```python
from build123d import *

# Parameters (mm, degrees)
CROQUIS1_RX                = 6.036526162
CROQUIS1_RY                = 3.070539463
CROQUIS1_RX_2              = 3.326417752
CROQUIS1_RY_2              = 2.687947262
SALIENTE_EXTRUIR2_DEPTH    = 5
CROQUIS7_W                 = 42.690533415
CROQUIS7_H                 = 0.890099334
CORTAR_EXTRUIR1_DEPTH      = 10
REDONDEO1_R                = 2.5
CROQUIS3_R                 = 1.1
SALIENTE_EXTRUIR3_DEPTH    = 11.5
SALIENTE_EXTRUIR4_START    = 11.5
CROQUIS6_R                 = 1.1
SALIENTE_EXTRUIR4_DEPTH    = 11.5
CORTAR_EXTRUIR2_DEPTH      = 61.024571756
CORTAR_EXTRUIR2_DEPTH_BACK = 61.024571756


with BuildPart() as part:
    # Croquis1 → Saliente-Extruir2 (new body)
    with BuildSketch(Plane.YZ):
        with BuildLine():
            Line((20.084653921, 11.717525193), (24.641633022, 14.68917463))
            ThreePointArc((24.641633022, 14.68917463), (27.816291871, 14.320547257), (28.034373421, 11.132007562))
            Line((28.034373421, 11.132007562), (20, 0))
            Line((20, 0), (20, -10))
            Line((20, -10), (15, -10))
            Line((15, -10), (15, -4.5))
            Line((15, -4.5), (3.5, -4.5))
            Line((3.5, -4.5), (3.5, -10))
            Line((3.5, -10), (-3.5, -10))
            Line((-3.5, -10), (-3.5, -4.5))
            Line((-3.5, -4.5), (-15, -4.5))
            Line((-15, -4.5), (-15, -10))
            Line((-15, -10), (-20, -10))
            Line((-20, -10), (-20, 0))
            Line((-20, 0), (-28.034373421, 11.132007562))
            ThreePointArc((-28.034373421, 11.132007562), (-27.816291871, 14.320547257), (-24.641633022, 14.68917463))
            Line((-24.641633022, 14.68917463), (-20.084653921, 11.717525193))
            ThreePointArc((-20.084653921, 11.717525193), (-14.865648019, 27.519606107), (0, 35))
            ThreePointArc((0, 35), (14.865648019, 27.519606107), (20.084653921, 11.717525193))
        make_face()
        with Locations(Location((-8.99716125, 20.68522558), (0, 0, 90))):
            Ellipse(CROQUIS1_RX, CROQUIS1_RY, mode=Mode.SUBTRACT)
        with Locations(Location((0, 6.95309076), (0, 0, -90))):
            Ellipse(CROQUIS1_RX_2, CROQUIS1_RY_2, mode=Mode.SUBTRACT)
        with Locations(Location((8.99716125, 20.68522558), (0, 0, 90))):
            Ellipse(CROQUIS1_RX, CROQUIS1_RY, mode=Mode.SUBTRACT)
    extrude(amount=SALIENTE_EXTRUIR2_DEPTH)

    # Croquis7 → Cortar-Extruir1 (cut)
    with BuildSketch(Plane.YZ):
        with Locations((-0.646243402, -10.047083115)):
            Rectangle(CROQUIS7_W, CROQUIS7_H)
    extrude(amount=CORTAR_EXTRUIR1_DEPTH, mode=Mode.SUBTRACT)

    # Redondeo1
    redondeo1_edges = [part.edges().sort_by_distance(p)[0] for p in [
        (0, 17.5, -9.602033448),
        (5, 17.5, -9.602033448),
        (0, 0, -9.602033448),
        (5, 0, -9.602033448),
        (0, -17.5, -9.602033448),
        (5, -17.5, -9.602033448),
    ]]
    fillet(redondeo1_edges, radius=REDONDEO1_R - 0.0001)  # a hair under: the kernel refuses the full size

    # Croquis3 → Saliente-Extruir3 (add)
    with BuildSketch(Plane(origin=(0, 3.5, 0), x_dir=(-1, 0, 0), z_dir=(0, 1, 0))):
        with Locations(Location((-2.5, -7.45, 0), (0, 0, 270))):
            Circle(CROQUIS3_R)
    extrude(amount=SALIENTE_EXTRUIR3_DEPTH)

    # Croquis6 → Saliente-Extruir4 (add)
    with BuildSketch(Plane.XZ.offset(3.5).offset(SALIENTE_EXTRUIR4_START)):
        with Locations(Location((2.5, -7.45, 0), (0, 0, 270))):
            Circle(CROQUIS6_R)
    extrude(amount=-SALIENTE_EXTRUIR4_DEPTH)

    # Croquis8 → Cortar-Extruir2 (cut, two sides: drawn at the far end of the back side and taken through both)
    with BuildSketch(Plane(origin=(0, 20, 0), x_dir=(-1, 0, 0), z_dir=(0, 1, 0)).offset(-CORTAR_EXTRUIR2_DEPTH_BACK)):
        with BuildLine():
            Line((-74.782541857, 59.609037795), (-6.886174559, -6.99410531))
            ThreePointArc((-6.886174559, -6.99410531), (-2.511263824, -8.781661023), (1.863646912, -6.99410531))
            Line((1.863646912, -6.99410531), (69.76001421, 59.609037795))
            Line((69.76001421, 59.609037795), (69.76001421, -130.610786238))
            Line((69.76001421, -130.610786238), (-74.782541857, -130.610786238))
            Line((-74.782541857, -130.610786238), (-74.782541857, 59.609037795))
        make_face()
    extrude(amount=CORTAR_EXTRUIR2_DEPTH + CORTAR_EXTRUIR2_DEPTH_BACK, mode=Mode.SUBTRACT)


solid = part.part
```
Build history of the part. All positions in model axes, mm. A direction names the side the tool comes from. Round coordinates to 2 decimals unless told otherwise and drop trailing zeros. Loops run counter-clockwise (first coordinate to the right, second up) from the corner with the lowest first, then second, coordinate; pieces in that order, holes last.
Item 1: Two-plate mould, pull along Y, no slides. Class faces 1 (the face through (2.46, 22.33, 13.18)), 2 (the face through (0, 0, 14)), 3 (the face through (2.46, -23.96, 5.49)), 4 (the face through (2, -9, -4.5)): released by +Y, released by -Y, zero draft, split by the parting line, or undercut.
Item 2: Saw through at C-C (y = -18). List the corners of the cut face in (x, z).
Item 3: Drill centre lines: line 1 along Y through (x, z) = (4.6, 16); line 2 along Z through (x, y) = (3.45, 10); line 3 along Y through (x, z) = (0.95, 21.5). Where is each one in solid material? Low to high.
Item 4: Saw through at A-A (y = -11). State how many separate pieces and enclosed holes the cut face has, then the cut area to 3 significant figures.
Item 5: Which spindle directions (+Z, -Z, +X, -X, +Y, -Y) get a long thin tool onto all of the face, cutting with end or side? Do faces 5 (the face through (2, 9, -4.5)), 6 (the face through (2, 15, -6)), 7 (the face through (0.1, -17.5, -7.8)), 8 (the face through (2, -20, -4)). Say none if no direction does.
Item 6: Pin check, flat tips, straight feed: P1, Ø1, axis at x = 4, y = 9.5, coming from the +Z side; P2, Ø2.5, axis at x = 2.5, y = 7, coming from the -Z side; P3, Ø2.5, axis at x = 1.5, z = -2.5, coming from the -Y side. Stop position of each tip, or through.
Worked answers:
1. face 1: undercut
1. face 2: zero draft
1. face 3: released by -Y
1. face 4: undercut
2. outline: (0, -7.1) arc R2.5 ccw to (0.36, -8.4) arc R6.25 ccw to (4.63, -8.41) arc R2.5 ccw to (5, -7.1) - (5, 22.73) - (0, 22.73) - close
3. line 1: y = -19.98 to -10.93, -7.06 to 7.06, 10.93 to 19.98
3. line 2: z = -8 to -6.9, -4.5 to 14.98, 26.39 to 31.71
3. line 3: y = -18.55 to -12.04, -5.95 to 5.95, 12.04 to 18.55
4. separate pieces: 3
4. enclosed holes: 0
4. area: 136 mm2
5. face 5: +X, -X
5. face 6: none
5. face 7: -Z, -X, +Y, -Y
5. face 8: -Z, +X, -X, -Y
6. P1: stops at z = 32.3
6. P2: stops at z = -8.55
6. P3: stops at y = -20
